Autodesk Inventor part; units mm, degrees
ref_plane "YZ Plane" through (0, 0, 0) normal (1, 0, 0) x (0, 1, 0)
ref_plane "XZ Plane" through (0, 0, 0) normal (0, 1, 0) x (-1, 0, 0)
ref_plane "XY Plane" through (0, 0, 0) normal (0, 0, 1) x (1, 0, 0)
sketch "Sketch1" plane through (0, 0, 0) normal (0, 0, 1) x (1, 0, 0)
  line L0 (24.4382, -12.9356) -> (-18.5618, -12.9356)
  line L1 (-18.5618, -12.9356) -> (-18.5618, 12.0644)
  line L2 (-18.5618, 12.0644) -> (24.4382, 12.0644)
  line L3 (24.4382, 12.0644) -> (24.4382, -12.9356)
  line L4 (-4.5618, -12.9356) -> (10.4382, -12.9356)
  line L5 (10.4382, -12.9356) -> (10.4382, -17.9356)
  line L6 (10.4382, -17.9356) -> (-4.5618, -17.9356)
  line L7 (-4.5618, -17.9356) -> (-4.5618, -12.9356)
  line L8 (-4.5618, 12.0644) -> (10.4382, 12.0644)
  line L9 (10.4382, 12.0644) -> (10.4382, 17.0644)
  line L10 (10.4382, 17.0644) -> (-4.5618, 17.0644)
  line L11 (-4.5618, 17.0644) -> (-4.5618, 12.0644)
  circle A0 centre (2.9382, -17.9356) radius 7.5
  circle A1 centre (2.9382, 17.0644) radius 7.5
  circle A2 centre (2.9382, -17.9356) radius 2.5
  circle A3 centre (2.9382, 17.0644) radius 2.5
  point P0 (0, 0)
  point P1 (-4.5618, -17.9356)
  dimension "d0" = 43
  dimension "d1" = 25
  dimension "d2" = 15
  dimension "d3" = 15
  dimension "d4" = 21.5
  dimension "d5" = 21.5
  dimension "d6" = 5
  dimension "d7" = 5
  dimension "d8" = 5
  dimension "d9" = 5
extrude "Extrusion1" add sketch "Sketch1" along normal blind 5 contours L0 A0 L1 L2 A1 L3 | L5 A0 L0 | A0 L6 A2 L0 | L0 A0 | A0 L6 A2 | L2 A1 L9 | A0 L7 L0 | A1 L2 | L2 A1 L10 A3 | L10 A3 A1 | L2 L11 A1
sketch "Sketch2" plane through (0, 0, 0) normal (0, 0, -1) x (-1, 0, 0)
  line L0 (18.5618, 12.0644) -> (18.5618, -12.9356)
  line L1 (-24.4382, -12.9356) -> (-24.4382, 12.0644)
  line L2 (18.5618, -12.9356) -> (-24.4382, -12.9356)
  line L3 (-24.4382, -12.9356) -> (-24.4382, -9.4356)
  line L4 (-24.4382, -9.4356) -> (18.5618, -9.4356)
  line L5 (18.5618, -9.4356) -> (18.5618, -12.9356)
  line L6 (-24.4382, 12.0644) -> (18.5618, 12.0644)
  line L7 (18.5618, 12.0644) -> (18.5618, 8.5644)
  line L8 (18.5618, 8.5644) -> (-24.4382, 8.5644)
  line L9 (-24.4382, 8.5644) -> (-24.4382, 12.0644)
  point P0 (0, 0)
  point P1 (-24.4382, 8.5644)
  point P2 (18.5618, -9.4356)
  dimension "d12" = 3.5
  dimension "d13" = 3.5
extrude "Extrusion2" add sketch "Sketch2" along normal blind 2 contours L0 L8 L1 L6 | L0 L2 L1 L4
sketch "Sketch3" plane through (0, 0, -2) normal (0, 0, -1) x (-1, 0, 0)
  line L0 (-24.4382, -12.9356) -> (18.5618, -12.9356)
  line L1 (-24.4382, -9.4356) -> (-24.4382, 8.5644)
  line L2 (18.5618, -12.9356) -> (-24.4382, -12.9356)
  line L3 (-24.4382, -12.9356) -> (-24.4382, -8.9356)
  line L4 (-24.4382, -8.9356) -> (18.5618, -8.9356)
  line L5 (18.5618, -8.9356) -> (18.5618, -12.9356)
  line L6 (-24.4382, 12.0644) -> (18.5618, 12.0644)
  line L7 (18.5618, 12.0644) -> (18.5618, 8.0644)
  line L8 (18.5618, 8.0644) -> (-24.4382, 8.0644)
  line L9 (-24.4382, 8.0644) -> (-24.4382, 12.0644)
  line L10 (-24.4382, -8.9356) -> (-22.4382, -8.9356)
  line L11 (-22.4382, -8.9356) -> (-22.4382, 8.0644)
  line L12 (-22.4382, 8.0644) -> (-24.4382, 8.0644)
  line L13 (-24.4382, 8.0644) -> (-24.4382, -8.9356)
  line L14 (-22.4382, -3.6663) -> (-20.4382, -3.6663)
  line L15 (-20.4382, -3.6663) -> (-20.4382, 2.486)
  line L16 (-20.4382, 2.486) -> (-22.4382, 2.486)
  line L17 (-22.4382, 2.486) -> (-22.4382, -3.6663)
  line L18 (18.5618, 12.0644) -> (-24.4382, 12.0644)
  point P0 (0, 0)
  dimension "d16" = 4
  dimension "d17" = 4
  dimension "d18" = 0
  dimension "d19" = 2
  dimension "d20" = 2
extrude "Extrusion3" add sketch "Sketch3" along normal blind 2
equation "\"d9\" = d8"
equation "\"d12\" = d13"
properties part number "RelayBracket"
Design review of the part built by this model. Coordinates are the model's own, in mm. A direction names the side the tool comes from. Coordinates: 2 decimals unless noted, no trailing zeros. Order: outer loops, then holes, each group sorted by start corner. A loop starts at its lowest first (then second) coordinate and runs counter-clockwise, first axis right, second up. Notation, with made-up numbers: (53, 56.25) - (80, 56.25) arc R30 ccw to (80, 78.25) - close; hole circle Ø5 at (52.25, -9). An arc over 180 degrees is marked (long way). Answer in a Markdown table with one row per item.
(1) The part is to be moulded in two halves that separate along Y. For faces 6 (the cylindrical face through (3.103, -25.434, 2.465)), 7 (the flat face through (10.438, -15, 2)), 8 (the flat face through (21, -3.666, -3)), 9 (the flat face through (3, 0, 0)), say which applies: released by +Y, released by -Y, zero draft, split by the parting line, or undercut.
Checked values:
| item | result |
|---|---|
| face 6 | released by -Y |
| face 7 | zero draft |
| face 8 | undercut |
| face 9 | undercut |
(2) Wall thickness on line 1 along Y through (x, z) = (5, -1.5); line 2 along Y through (x, z) = (4, -2.25); line 3 along Y through (x, z) = (3.5, 4.5): over which ranges is each line inside the solid? List them lowest first. Write a range as from..to.
Checked values:
| item | result |
|---|---|
| line 1 | -12.94..-9.44, 8.56..12.06 |
| line 2 | -12.94..-8.94, 8.06..12.06 |
| line 3 | -25.41..-20.37, -15.5..14.63, 19.5..24.54 |
(3) Consider section A-A on y = 6. State the section outline as (x, z) points, plus the area to 3 significant figures.
Checked values:
| item | result |
|---|---|
| outline | (-18.56, 0) - (24.44, 0) - (24.44, 5) - (-18.56, 5) - close; (22.44, -4) - (24.44, -4) - (24.44, -2) - (22.44, -2) - close |
| area | 219 mm^2 |
(4) For faces 1 (the flat face through (-4.562, 15, 2)), 2 (the flat face through (21, 0, -2)), 3 (the flat face through (2, -8.936, -3)), 4 (the flat face through (3, 20, 0)), 5 (the cylindrical face through (2.613, 14.586, 2.465)), list the 3-axis set-ups (+Z, -Z, +X, -X, +Y, -Y) from which the entire face can be reached by the end or side of a thin tool; tool diameter is ignored.
Checked values:
| item | result |
|---|---|
| face 1 | +Z, -Z, -X, +Y |
| face 2 | +X, -X |
| face 3 | -Z, -X |
| face 4 | -Z, +X, -X, +Y |
| face 5 | +Z, -Z |
(5) Consider section D-D on x = 1. State the section outline as (y, z) points, plus the area to 3 significant figures.
Checked values:
| item | result |
|---|---|
| outline | (-25.18, 0) - (-19.51, 0) - (-19.51, 5) - (-25.18, 5) - close; (-16.36, 0) - (-12.94, 0) - (-12.94, -4) - (-8.94, -4) - (-8.94, -2) - (-9.44, -2) - (-9.44, 0) - (8.56, 0) - (8.56, -2) - (8.06, -2) - (8.06, -4) - (12.06, -4) - (12.06, 0) - (15.49, 0) - (15.49, 5) - (-16.36, 5) - close; (18.64, 0) - (24.31, 0) - (24.31, 5) - (18.64, 5) - close |
| area | 246 mm^2 |
(6) Clearance check with flat-ended pins moving along their axes: pin 1 (1.6 mm diameter, centred on y = -5.5, z = -3.5, fed in from -X); pin 2 (1.5 mm diameter, centred on y = 14, z = 2.5, fed in from -X); pin 3 (1 mm diameter, centred on x = 19, z = 3, fed in from +Y). State where each tip first meets the part, or that it passes through.
Checked values:
| item | result |
|---|---|
| pin 1 | x = 22.44 |
| pin 2 | x = -4.56 |
| pin 3 | y = 12.06 |
(7) Consider section B-B on z = -1.25. State the section outline as (x, y) points.
Checked values:
| item | result |
|---|---|
| outline | (-18.56, -12.94) - (24.44, -12.94) - (24.44, -9.44) - (-18.56, -9.44) - close; (-18.56, 8.56) - (24.44, 8.56) - (24.44, 12.06) - (-18.56, 12.06) - close |
(8) Consider section C-C on z = 3.5. State the section outline as (x, y) points.
Checked values:
| item | result |
|---|---|
| outline | (-18.56, -12.94) - (-4.56, -12.94) - (-4.56, -17.94) arc R7.5 ccw to (10.44, -17.94) - (10.44, -12.94) - (24.44, -12.94) - (24.44, 12.06) - (10.44, 12.06) - (10.44, 17.06) arc R7.5 ccw to (-4.56, 17.06) - (-4.56, 12.06) - (-18.56, 12.06) - close; hole circle Ø5 at (2.94, -17.94); hole circle Ø5 at (2.94, 17.06) |
